Source: CAD feature listing. Evaluate the final solid. Frame: model axes, mm. Face numbers are marked on the shaded views. A direction names the side the tool comes from. Give positions to 0.01 mm unless a question says otherwise; leave off trailing zeros. Loops run counter-clockwise (first coordinate to the right, second up) from the corner with the lowest first, then second, coordinate; pieces in that order, holes last. Notation, with made-up numbers: (28.25, 77) -> (50.25, 77) arc R25 cw to (50.25, 113) -> close; hole circle Ø1 at (31, -4.5). An arc over 180 degrees is marked (long way). Return JSON: item names as keys, results as strings. Group by question number.
(1) Cut plane B-B on z = 6.75. Return loops of the section in (x, y).
(2) Cut plane C-C on x = -7.5. Return loops of the section in (y, z).
(3) Cut plane D-D on y = 11. Return loops of the section in (x, z).
(4) Pin query (flat end, axial travel): pin 1 (2 mm diameter, centred on y = 2, z = 10.5, fed in from -X); pin 2 (3 mm diameter, centred on x = -29.5, z = 7.5, fed in from +Y); pin 3 (8 mm diameter, centred on x = -62, z = 7.5, fed in from -Y); pin 4 (4 mm diameter, centred on y = 3.5, z = 10, fed in from -X). Return the tip coordinate at first contact, or that it passes through.
(5) Cut plane A-A on y = 7.5. Return loops of the section in (x, z).
(6) Ray query, line 1 (Y direction, x = -7.5, z = 8.75); line 2 (Y direction, x = -34.5, z = 13); line 3 (X direction, y = 14.5, z = 1.25). Return the intervals inside material, ascending. Write a range as from..to.
(7) Access query for the marked faces 1, 2 and 3. Directions: +Z, -Z, +X, -X, +Y, -Y. A direction counts if a zero-diameter tool reaches every point of the face in a straight line with its end or side. Return the directions, or none.
```python
from build123d import *

# Parameters (mm, degrees)
AUFSATZ_LINEAR_AUSTRAGEN1_DEPTH = 18
SKIZZE2_R                       = 2.5
SCHNITT_LINEAR_AUSTRAGEN1_DEPTH = 19
VERRUNDUNG1_R                   = 5


with BuildPart() as part:
    # Skizze1 → Aufsatz-Linear austragen1 (new body)
    with BuildSketch(Plane.XY):
        Polygon((0, 0), (-15, 0), (-15, 5), (-75, 5), (-75, 10), (-15, 10), (-15, 15), (0, 15), align=None)
    extrude(amount=AUFSATZ_LINEAR_AUSTRAGEN1_DEPTH)

    # Skizze2 → Schnitt-Linear austragen1 (cut, through all)
    with BuildSketch(Plane.XY.offset(18)):
        with Locations((-7.5, 7.5)):
            Circle(SKIZZE2_R)
    extrude(amount=-SCHNITT_LINEAR_AUSTRAGEN1_DEPTH, mode=Mode.SUBTRACT)

    # Verrundung1
    verrundung1_edges = [part.edges().sort_by_distance(p)[0] for p in [
        (0, 0, 9),
    ]]
    fillet(verrundung1_edges, radius=VERRUNDUNG1_R)


solid = part.part
```
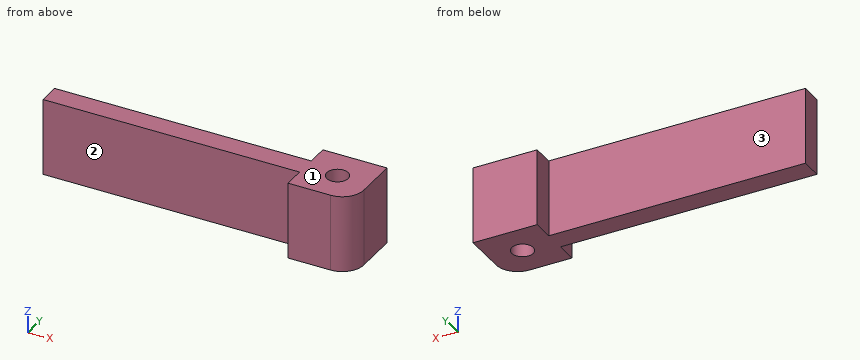
Answers:
{
 "1": {"outline": "(-75, 5) -> (-15, 5) -> (-15, 0) -> (-5, 0) arc R5 ccw to (0, 5) -> (0, 15) -> (-15, 15) -> (-15, 10) -> (-75, 10) -> close; hole circle Ø5 at (-7.5, 7.5)"},
 "2": {"outline": "(0, 0) -> (5, 0) -> (5, 18) -> (0, 18) -> close; (10, 0) -> (15, 0) -> (15, 18) -> (10, 18) -> close"},
 "3": {"outline": "(-15, 0) -> (0, 0) -> (0, 18) -> (-15, 18) -> close"},
 "4": {"pin 1": "x = -15", "pin 2": "y = 10", "pin 3": "y = 5", "pin 4": "x = -75"},
 "5": {"outline": "(-75, 0) -> (-10, 0) -> (-10, 18) -> (-75, 18) -> close; (-5, 0) -> (0, 0) -> (0, 18) -> (-5, 18) -> close"},
 "6": {"line 1": "0..5, 10..15", "line 2": "5..10", "line 3": "-15..0"},
 "7": {"face 1": "+Z, +X, -X, +Y, -Y", "face 2": "+Z, -Z, -X, -Y", "face 3": "+Z, -Z, -X, +Y"}
}
